Autodesk Inventor part; units mm, degrees
ref_plane "YZ Plane" through (0, 0, 0) normal (1, 0, 0) x (0, 1, 0)
ref_plane "XZ Plane" through (0, 0, 0) normal (0, 1, 0) x (-1, 0, 0)
ref_plane "XY Plane" through (0, 0, 0) normal (0, 0, 1) x (1, 0, 0)
sketch "Sketch1" plane through (0, 0, 0) normal (0, 0, 1) x (1, 0, 0)
  line L0 (-12.1708, 16.0073) -> (13.2292, 16.0073)
  line L1 (13.2292, 16.0073) -> (13.2292, -34.7927)
  line L2 (13.2292, -34.7927) -> (-12.1708, -34.7927)
  line L3 (-12.1708, -34.7927) -> (-12.1708, 16.0073)
  line L4 (11.9592, 14.7373) -> (-10.9008, 14.7373)
  line L5 (-10.9008, 14.7373) -> (-10.9008, -33.5227)
  line L6 (-10.9008, -33.5227) -> (11.9592, -33.5227)
  line L7 (11.9592, -33.5227) -> (11.9592, 14.7373)
  point P0 (0, 0)
  dimension "d0" = 25.4
  dimension "d1" = 50.8
  dimension "d2" = 1.27
extrude "Extrusion1" add sketch "Sketch1" along normal blind 457.2
sketch "Sketch2" plane through (-12.1708, 16.0073, 0) normal (0, 1, 0) x (1, 0, 0)
  circle A0 centre (12.7, -12.7) radius 1.7272
  line L0 (25.4, 0) -> (0, 0)
  line L1 (0, 0) -> (0, -457.2)
  point P0 (12.1708, 0)
  dimension "d5" = 3.4544
  dimension "d6" = 12.7
  dimension "d7" = 12.7
extrude "Extrusion2" cut sketch "Sketch2" against normal through all
pattern_linear "Rectangular Pattern1" count 46 spacing 25.4 along (0, 0, 1) of "Extrusion2"
sketch "Sketch5" plane through (13.2292, -34.7927, 0) normal (1, 0, 0) x (0, 0, -1)
  circle A0 centre (-444.5, 25.4) radius 2.3813
  circle A1 centre (-431.8, 25.4) radius 2.3813
  line L0 (-444.5, 25.4) -> (-419.1, 25.4)
  line L1 (0, 0) -> (-457.2, 0)
  line L2 (-457.2, 0) -> (-457.2, 50.8)
  circle A2 centre (-38.1, 25.4) radius 2.3813
  circle A3 centre (-25.4, 25.4) radius 2.3813
  circle A4 centre (-12.7, 25.4) radius 2.3813
  line L3 (-38.1, 25.4) -> (-12.7, 25.4)
  line L4 (0, 0) -> (0, 50.8)
  point P0 (0, 34.7927)
  dimension "d40" = 4.7625
  dimension "d41" = 25.4
  dimension "d42" = 25.4
  dimension "d43" = 12.7
  dimension "d44" = 4.7625
  dimension "d45" = 25.4
  dimension "d46" = 25.4
  dimension "d47" = 12.7
extrude "Extrusion5" cut sketch "Sketch5" against normal through all
equation "\"d3\" = d13"
equation "\"d10\" = d14"
equation "\"d13\" = 457.2"
equation "\"d14\" = d13"
properties part number "Long bar 4- VersaFrame"
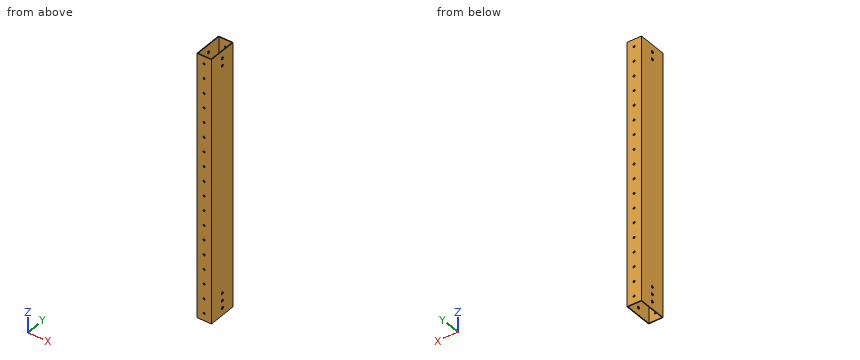
Read the model definition and answer for the solid it produces. Units are mm, in the model's axes. Round coordinates to 2 decimals unless told otherwise and drop trailing zeros. Write each loop counter-clockwise with the first axis right and the second up, starting at its lowest first coordinate (ties: lowest second). Pieces come first, ordered by that corner, then holes.
Q1. A flat-ended cylindrical pin translates along its axis: P1, Ø2, axis at x = 0.53, z = 444.5, coming from the +Y side. Find the tip coordinate at first contact, or state that the pin passes through.
Values:
P1: passes through
Q2. Find section C-C on z = 378. Determine the outline of the cut face in (x, y).
Values:
outline: (-12.17, -34.79) - (13.23, -34.79) - (13.23, 16.01) - (-12.17, 16.01) - close; hole (-10.9, -33.52) - (11.96, -33.52) - (11.96, 14.74) - (-10.9, 14.74) - close
Q3. Find section A-A on y = -15.5. Determine the outline of the cut face in (x, z), and give its area (3 significant figures).
Values:
outline: (-12.17, 0) - (-10.9, 0) - (-10.9, 457.2) - (-12.17, 457.2) - close; (11.96, 0) - (13.23, 0) - (13.23, 457.2) - (11.96, 457.2) - close
area: 1,160 mm2
Q4. Straight lines are drawn through the part: line 1 (Y direction, x = -10, z = 230); line 2 (X direction, y = -34.1, z = 419.1); line 3 (X direction, y = -12, z = 374). For each, find the intervals that lie inside material, in ascending order.
Values:
line 1: y = -34.79 to -33.52, 14.74 to 16.01
line 2: x = -12.17 to -1.2, 2.26 to 13.23
line 3: x = -12.17 to -10.9, 11.96 to 13.23
Q5. Find section B-B on x = 8.25. Determine the outline of the cut face in (y, z).
Values:
outline: (-34.79, 0) - (-33.52, 0) - (-33.52, 457.2) - (-34.79, 457.2) - close; (14.74, 0) - (16.01, 0) - (16.01, 457.2) - (14.74, 457.2) - close
